from build123d import *

# Parameters (mm, degrees)
BASE_FLANGE1_DEPTH                                = 2
SKETCH7_R                                         = 2
CUT_EXTRUDE1_DEPTH                                = 2
CSK_FOR_4_FLAT_HEAD_MACHINE_SCREW_100_D           = 3.2639
CSK_FOR_4_FLAT_HEAD_MACHINE_SCREW_100_DEPTH       = 2
CSK_FOR_4_FLAT_HEAD_MACHINE_SCREW_100_CSINK_D     = 5.715
CSK_FOR_4_FLAT_HEAD_MACHINE_SCREW_100_CSINK_ANGLE = 100
CSK_FOR_4_FLAT_HEAD_MACHINE_SCREW_100_TIP         = 0.980574487


# Sheet-metal steps are written as plain solids
with BuildPart() as part:
    # Sketch2 → Base-Flange1 (new body)
    with BuildSketch(Plane(origin=(0, 0, 0), x_dir=(1, 0, 0), z_dir=(0, 1, 0))):
        with BuildLine():
            Line((-29.4, -3.310589071), (-34.53, -3.310589071))
            ThreePointArc((-34.53, -3.310589071), (-36.836910234, -6.744553073), (-40.41, -8.829492668))
            Line((-40.41, -8.829492668), (-40.41, -22.72))
            Line((-40.41, -22.72), (-40.41, -47.72))
            Line((-40.41, -47.72), (-30.41, -47.72))
            Line((-30.41, -47.72), (-30.41, -22.72))
            Line((-30.41, -22.72), (22.95, -22.72))
            Line((22.95, -22.72), (22.95, -7.25))
            ThreePointArc((22.95, -7.25), (19.171063031, -6.187255885), (16.5, -3.310589071))
            ThreePointArc((16.5, -3.310589071), (11.475, -0.241513115), (6.45, -3.310589071))
            ThreePointArc((6.45, -3.310589071), (0, -7.25), (-6.45, -3.310589071))
            ThreePointArc((-6.45, -3.310589071), (-11.475, -0.241513115), (-16.5, -3.310589071))
            ThreePointArc((-16.5, -3.310589071), (-22.95, -7.25), (-29.4, -3.310589071))
        make_face()
    extrude(amount=-BASE_FLANGE1_DEPTH)

    # Sketch7 → Cut-Extrude1 (cut)
    with BuildSketch(Plane(origin=(0, 0, 0), x_dir=(1, 0, 0), z_dir=(0, 1, 0))):
        with Locations(Location((-35.41, -41.22, 0), (0, 0, 270))):
            Circle(SKETCH7_R)
        with Locations(Location((-35.41, -31.72, 0), (0, 0, 270))):
            Circle(SKETCH7_R)
    extrude(amount=-CUT_EXTRUDE1_DEPTH, mode=Mode.SUBTRACT)

    # CSK for #4 Flat Head Machine Screw (100)1
    with Locations(Plane(origin=(0, 0, 0), x_dir=(1, 0, 0), z_dir=(0, 1, 0))):
        with Locations((-19.29, -14.86), (1.83, -14.86)):
            CounterSinkHole(CSK_FOR_4_FLAT_HEAD_MACHINE_SCREW_100_D / 2, CSK_FOR_4_FLAT_HEAD_MACHINE_SCREW_100_CSINK_D / 2, depth=CSK_FOR_4_FLAT_HEAD_MACHINE_SCREW_100_DEPTH, counter_sink_angle=CSK_FOR_4_FLAT_HEAD_MACHINE_SCREW_100_CSINK_ANGLE)
            with Locations((0, 0, -(CSK_FOR_4_FLAT_HEAD_MACHINE_SCREW_100_DEPTH + CSK_FOR_4_FLAT_HEAD_MACHINE_SCREW_100_TIP / 2))):  # 118° drill point
                Cone(0, CSK_FOR_4_FLAT_HEAD_MACHINE_SCREW_100_D / 2, CSK_FOR_4_FLAT_HEAD_MACHINE_SCREW_100_TIP, mode=Mode.SUBTRACT)


solid = part.part
Model file for the job. Use its own axes, mm. A direction names the side the tool comes from. Coordinates: 2 decimals unless noted, no trailing zeros. Write each loop counter-clockwise with the first axis right and the second up, starting at its lowest first coordinate (ties: lowest second). Pieces come first, ordered by that corner, then holes. Notation, with made-up numbers: (79.25, 6) -> (108.25, 6) arc R9 cw to (108.25, 12) -> close; hole circle Ø8 at (40.5, -9). An arc over 180 degrees is marked (long way). One line per item, written item: value. Start each with the question number.
1) Which spindle directions (+Z, -Z, +X, -X, +Y, -Y) get a long thin tool onto all of the face, cutting with end or side? Do faces 4 (the face through (-30.41, -1, 35)), 5 (the face through (-36.79, -0.99, 6.7)). Say none if no direction does.
2) Probe probe 1 along X at (y, z) = (-1.15, 41.22); probe 2 along X at (y, z) = (-1.3, 3.5) (3 decimals); probe 3 along X at (y, z) = (-1.5, 5). List the from-to ranges inside material, lowest first.
3) Slice it at A-A on z = 14.86. Write the cut outline in (x, y), then the cut area to 3 significant figures.
4) Slice it at B-B on z = 41.22. Write the cut outline in (x, y).
5) Pull direction X, two halves, no side cores. Call faces 1 (the face through (-35, -1, 47.72)), 2 (the face through (22.95, -1, 15)), 3 (the face through (11.562, -0.986, 0.242)): +X half, -X half, draft (parallel to the pull), parting line (faces both ways), or undercut.
6) Slice it at D-D on x = -19.29. Write the cut outline in (y, z), then the cut area to 3 significant figures.
7) Slice it at C-C on x = -35.41. Write the cut outline in (y, z), then the cut area to 3 significant figures.
8) Flat gauge pin, fed straight in: pin 1 Ø1 at (x, y) = (12.5, -1.5) entering from -Z. Where does the tip first touch, or does it go through?
Answers follow:
1. face 4: +Z, +X, +Y, -Y
1. face 5: -Z, -X, +Y, -Y
2. probe 1: -40.41 to -37.41, -33.41 to -30.41
2. probe 2: -34.605 to -29.299, -16.601 to -6.349, 6.349 to 16.601
2. probe 3: -35.39 to -28.2, -17.7 to -5.25, 5.25 to 17.7
3. outline: (-40.41, -2) -> (-20.92, -2) -> (-20.92, -1.03) -> (-22.15, 0) -> (-40.41, 0) -> close; (-17.66, -2) -> (0.2, -2) -> (0.2, -1.03) -> (-1.03, 0) -> (-16.43, 0) -> (-17.66, -1.03) -> close; (3.46, -2) -> (22.95, -2) -> (22.95, 0) -> (4.69, 0) -> (3.46, -1.03) -> close
3. area: 111 mm2
4. outline: (-40.41, -2) -> (-37.41, -2) -> (-37.41, 0) -> (-40.41, 0) -> close; (-33.41, -2) -> (-30.41, -2) -> (-30.41, 0) -> (-33.41, 0) -> close
5. face 1: draft
5. face 2: +X half
5. face 3: undercut
6. outline: (-2, 6.26) -> (0, 6.26) -> (0, 12) -> (-1.03, 13.23) -> (-2, 13.23) -> close; (-2, 16.49) -> (-1.03, 16.49) -> (0, 17.72) -> (0, 22.72) -> (-2, 22.72) -> close
6. area: 25.1 mm2
7. outline: (-2, 5.04) -> (0, 5.04) -> (0, 29.72) -> (-2, 29.72) -> close; (-2, 33.72) -> (0, 33.72) -> (0, 39.22) -> (-2, 39.22) -> close; (-2, 43.22) -> (0, 43.22) -> (0, 47.72) -> (-2, 47.72) -> close
7. area: 69.4 mm2
8. pin 1: z = 0.27
